Source: CAD feature listing. Evaluate the final solid. Frame: model axes, mm. Face numbers are marked on the shaded views. Round coordinates to 2 decimals unless told otherwise and drop trailing zeros. Order: outer loops, then holes, each group sorted by start corner. A loop starts at its lowest first (then second) coordinate and runs counter-clockwise, first axis right, second up. Notation, with made-up numbers: (70, 18.5) -> (129, 18.5) arc R19 cw to (129, 39.5) -> close; hole circle Ø1 at (45, 69). An arc over 180 degrees is marked (long way). One line per item, written item: value. Start each with the question number.
1) Mould query, pull axis Z, two halves, no side actions, for the marked faces 1, 2 and 3. Classes: pulls with the +Z half, pulls with the -Z half, needs draft (parallel to the pull), parting line crosses it, or undercut.
2) Pin query (flat end, axial travel): P1, Ø6, axis at x = -47, z = 0, coming from the +Y side; P2, Ø1.9, axis at y = 2.5, z = -1.5, coming from the +X side; P3, Ø6.5, axis at x = 20, z = 1.5, coming from the -Y side; P4, Ø6, axis at x = -27, z = 7, coming from the -Y side. Return the tip coordinate at first contact, or that it passes through.
3) Ray query, L1, parallel to Y at x = -57, z = 3.5; L2, parallel to Z at x = -48, y = 3.25; L3, parallel to X at y = 9.75, z = -0.25. Return the intervals inside material, ascending.
4) Section D-D (x = -46). Return the cut outline in (y, z).
5) Section A-A (y = 2.5). Return the cut outline in (x, z) (3 decimals), and give its area (3 significant figures).
6) Section B-B (x = 17). Return the cut outline in (y, z) (3 decimals), and give its area (3 significant figures).
7) Section C-C (z = -2.75). Return the cut outline in (x, y), and give its area (3 significant figures).
Autodesk Inventor part; units mm, degrees
ref_plane "YZ Plane" through (0, 0, 0) normal (1, 0, 0) x (0, 1, 0)
ref_plane "XZ Plane" through (0, 0, 0) normal (0, 1, 0) x (-1, 0, 0)
ref_plane "XY Plane" through (0, 0, 0) normal (0, 0, 1) x (1, 0, 0)
sketch "Sketch1" plane through (0, 0, 0) normal (0, 1, 0) x (-1, 0, 0)
  line L0 (-38.1, 9.525) -> (38.1, 9.525)
  line L1 (38.1, 9.525) -> (38.1, -9.525)
  line L2 (38.1, -9.525) -> (-38.1, -9.525)
  line L3 (-38.1, -9.525) -> (-38.1, 9.525)
  line L4 (38.1, 6.223) -> (63.246, 6.223)
  line L5 (63.246, 6.223) -> (63.246, -6.223)
  line L6 (63.246, -6.223) -> (38.1, -6.223)
  line L7 (38.1, -6.223) -> (38.1, 6.223)
  point P0 (0, 0)
  point P1 (38.1, 0)
  dimension "d0" = 76.2
  dimension "d1" = 19.05
  dimension "d2" = 9.525
  dimension "d3" = 38.1
  dimension "d4" = 25.146
  dimension "d5" = 12.446
  dimension "d6" = 6.223
extrude "Extrusion1" add sketch "Sketch1" along normal blind 6.35
sketch "Sketch2" plane through (38.1, 0, 9.525) normal (1, 0, 0) x (0, 0, -1)
  line L0 (0, 0) -> (19.05, 0)
  line L1 (19.05, 0) -> (19.05, 6.35)
  line L2 (0, 6.35) -> (19.05, 6.35)
  line L3 (0, 0) -> (0, 6.35)
  line L4 (19.05, 0) -> (19.05, 6.35)
  line L5 (0, 0) -> (0, 6.35)
  arc A0 (19.05, 6.35) -> (0, 6.35) centre (9.525, 0) ccw
  point P0 (9.525, 0)
extrude "Extrusion2" add sketch "Sketch2" against normal blind 76.2 contours A0 L2
sketch "Sketch3" plane through (0, 0, 0) normal (0, -1, 0) x (1, 0, 0)
  line L0 (38.1, 9.525) -> (38.1, -9.525)
  line L1 (-38.1, 9.525) -> (38.1, 9.525)
  line L2 (-38.1, 6.223) -> (-38.1, 9.525)
  line L3 (-63.246, 6.223) -> (-38.1, 6.223)
  line L4 (-63.246, -6.223) -> (-63.246, 6.223)
  line L5 (-38.1, -6.223) -> (-63.246, -6.223)
  line L6 (-38.1, -9.525) -> (-38.1, -6.223)
  line L7 (38.1, -9.525) -> (-38.1, -9.525)
  line L8 (38.1, -9.525) -> (38.1, 9.525)
  line L9 (38.1, 6.35) -> (12.7, 6.35)
  line L10 (12.7, 6.35) -> (12.7, -6.35)
  line L11 (12.7, -6.35) -> (38.1, -6.35)
  line L12 (38.1, -6.35) -> (38.1, 6.35)
  point P0 (0, 0)
  point P1 (38.1, 0)
  dimension "d11" = 12.7
  dimension "d12" = 12.446
  dimension "d13" = 6.35
  dimension "d14" = 25.4
extrude "Extrusion3" cut sketch "Sketch3" against normal blind 6.35 contours L0 L11 L10 L9
sketch "Sketch4" plane through (0, 6.35, 0) normal (0, 1, 0) x (1, 0, 0)
  line L0 (-38.1, -6.223) -> (-38.1, 6.223)
  line L1 (-38.1, 6.223) -> (-63.246, 6.223)
  line L2 (-63.246, 6.223) -> (-63.246, -6.223)
  line L3 (-63.246, -6.223) -> (-38.1, -6.223)
  point P0 (0, 0)
extrude "Extrusion4" cut sketch "Sketch4" against normal blind 0.254
properties part number "Part_3_hand_extention"
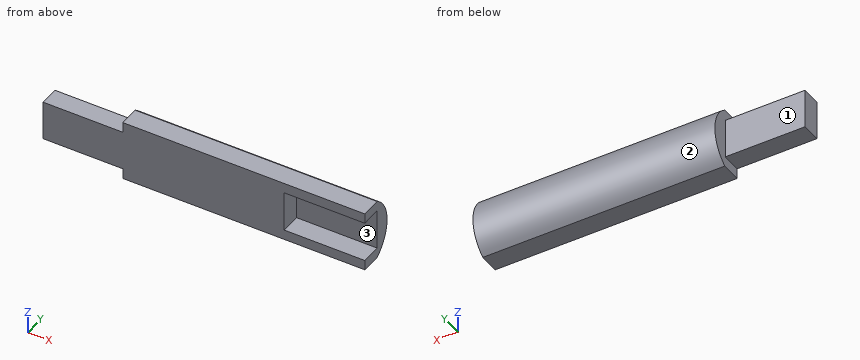
Findings:
1. face 1: needs draft
1. face 2: parting line crosses it
1. face 3: undercut
2. P1: y = 6.1
2. P2: x = 12.7
2. P3: y = 6.35
2. P4: y = 0
3. L1: 0 to 6.1
3. L2: -6.22 to 6.22
3. L3: -38.1 to 38.1
4. outline: (0, -6.22) -> (6.1, -6.22) -> (6.1, 6.22) -> (0, 6.22) -> close
5. outline: (-63.246, -6.223) -> (-38.1, -6.223) -> (-38.1, -9.525) -> (38.1, -9.525) -> (38.1, -6.35) -> (12.7, -6.35) -> (12.7, 6.35) -> (38.1, 6.35) -> (38.1, 9.525) -> (-38.1, 9.525) -> (-38.1, 6.223) -> (-63.246, 6.223) -> close
5. area: 1,440 mm2
6. outline: (0, -9.525) -> (6.35, -9.525) arc R11.448 ccw to (6.35, 9.525) -> (0, 9.525) -> (0, 6.35) -> (6.35, 6.35) -> (6.35, -6.35) -> (0, -6.35) -> close
6. area: 109 mm2
7. outline: (-63.25, 0) -> (12.7, 0) -> (12.7, 6.35) -> (38.1, 6.35) -> (38.1, 11.11) -> (-38.1, 11.11) -> (-38.1, 6.1) -> (-63.25, 6.1) -> close
7. area: 839 mm2
